Autodesk Inventor part; units mm, degrees
ref_plane "YZ Plane" through (0, 0, 0) normal (1, 0, 0) x (0, 1, 0)
ref_plane "XZ Plane" through (0, 0, 0) normal (0, 1, 0) x (-1, 0, 0)
ref_plane "XY Plane" through (0, 0, 0) normal (0, 0, 1) x (1, 0, 0)
sketch "Skizze1" plane through (0, 0, 0) normal (0, 0, 1) x (1, 0, 0)
  circle A0 centre (0.0001, -0.0022) radius 3.9802
  circle A1 centre (-8.37, 7.9978) radius 1.4
  circle A2 centre (8.3745, -8.0022) radius 1.4
  line L0 (-9.5383, 7.2264) -> (-3.2198, -2.3418)
  line L1 (-7.6522, 9.1998) -> (1.8915, 3.4999)
  line L2 (9.5428, -7.2307) -> (3.3215, 2.191)
  line L3 (-1.8517, -3.5253) -> (7.6567, -9.2041)
  point P0 (0, 0)
extrude "Extrusion1" add sketch "Skizze1" along normal blind 2
sketch "Skizze2" plane through (0, 0, 2) normal (0, 0, 1) x (1, 0, 0)
  arc A0 (-7.6522, 9.1998) -> (-9.5383, 7.2264) centre (-8.37, 7.9978) ccw
  line L0 (-9.5383, 7.2264) -> (-3.2198, -2.3418)
  arc A1 (-3.2198, -2.3418) -> (-1.8517, -3.5253) centre (0.0001, -0.0022) ccw
  line L1 (-1.8517, -3.5253) -> (7.6567, -9.2041)
  arc A2 (7.6567, -9.2041) -> (9.5428, -7.2307) centre (8.3745, -8.0022) ccw
  line L2 (9.5428, -7.2307) -> (3.3215, 2.191)
  arc A3 (3.3215, 2.191) -> (1.8915, 3.4999) centre (0.0001, -0.0022) ccw
  line L3 (1.8915, 3.4999) -> (-7.6522, 9.1998)
  arc A4 (-6.6267, 10.9169) -> (-11.2072, 6.1243) centre (-8.37, 7.9978) ccw
  line L4 (-11.2072, 6.1243) -> (-4.8666, -3.4774)
  arc A5 (-4.8666, -3.4774) -> (-2.8352, -5.2674) centre (0.0001, -0.0022) ccw
  line L5 (-2.8352, -5.2674) -> (6.6312, -10.9212)
  arc A6 (6.6312, -10.9212) -> (11.2118, -6.1287) centre (8.3745, -8.0022) ccw
  line L6 (11.2118, -6.1287) -> (4.9905, 3.2931)
  arc A7 (4.9905, 3.2931) -> (2.8837, 5.2369) centre (0.0001, -0.0022) ccw
  line L7 (2.8837, 5.2369) -> (-6.6267, 10.9169)
  point P0 (0, 0)
  dimension "d2" = 2
extrude "Extrusion2" add sketch "Skizze2" against normal up to surface (2 mm away)
sketch "Skizze3" plane through (0, 0, 2) normal (0, 0, 1) x (1, 0, 0)
  circle A0 centre (0.0001, -0.0022) radius 3.9802
  circle A1 centre (-8.37, 7.9978) radius 1.4
  circle A2 centre (8.3745, -8.0022) radius 1.4
  circle A3 centre (0.0001, -0.0022) radius 3.35
  point P0 (0, 0)
  dimension "d5" = 6.7
extrude "Extrusion3" cut sketch "Skizze3" against normal through all contours A1 | A2 | A3
sketch "Skizze4" plane through (0, 0, 2) normal (0, 0, 1) x (1, 0, 0)
  circle A0 centre (-8.37, 7.9978) radius 1.4
  circle A1 centre (8.3745, -8.0022) radius 1.4
  point P0 (0, 0)
hole "Bohrung1" at (-8.37, 7.9978, 2) at (8.3745, -8.0022, 2) direction (0, 0, -1) diameter 2.8 end through all
chamfer "Fase1" distance 1 angle 45 1 edges at (-3.3499, -0.0022, 2)
properties part number "IM_Lensholder_macroscope"
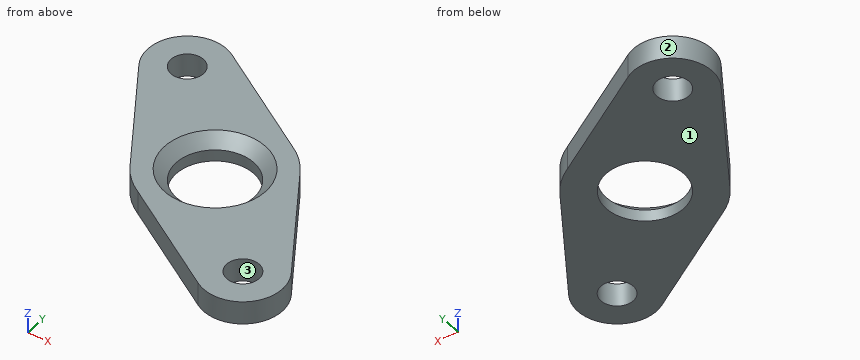
Could you check a few things on this model? Use its own coordinates, in mm. Face numbers are marked on the shaded views. Give positions to 0.01 mm unless a question says otherwise; leave off trailing zeros. Order: outer loops, then holes, each group sorted by start corner. A loop starts at its lowest first (then second) coordinate and runs counter-clockwise, first axis right, second up. Notation, with made-up numbers: (-29.75, 80.5) - (22.25, 80.5) arc R28 cw to (22.25, 119.5) - close; hole circle Ø6 at (31.25, 65). An arc over 180 degrees is marked (long way). Return JSON: item names as keys, results as strings. Group by question number.
Q1. Thinking about a two-plate mould opening in X: for the marked faces 1, 2 and 3, which applies, pulls with the +X half, pulls with the -X half, needs draft (parallel to the pull), parting line crosses it, or undercut?
Q2. Suppose I cut it at C-C, the plane x = -6. Please give me the cut outline in (y, z), and give its area (3 significant figures).
Q3. Suppose I cut it at D-D, the plane y = 5.5. Please give me the cut outline in (x, z).
Q4. Please list where these lines run through material, in increasing order: line 1 along Y through (x, z) = (2.5, 1.45); line 2 along X through (y, z) = (8.5, 0.85); line 3 along X through (y, z) = (3, 1.1). Write a range as [from, to].
Q5. Will these pins go through, and if not, where does the flat tip stop? pin 1 Ø3.5 at (x, y) = (8.37, -8) entering from -Z; pin 2 Ø1 at (y, z) = (7.5, 1.5) entering from +X.
Q6. Suppose I cut it at A-A, the plane z = 1.35. Please give me the cut outline in (x, y), and give its area (3 significant figures).
Q7. Suppose I cut it at B-B, the plane x = -8.37. Please give me the cut outline in (y, z).
Resolved:
{
 "1": {"face 1": "needs draft", "face 2": "parting line crosses it", "face 3": "undercut"},
 "2": {"outline": "(-1.76, 0) - (10.54, 0) - (10.54, 2) - (-1.76, 2) - close", "area": "24.6 mm2"},
 "3": {"outline": "(-10.79, 0) - (2.44, 0) - (2.44, 2) - (-10.79, 2) - close"},
 "4": {"line 1": "y = [-8.45, -2.86], [2.86, 5.47]", "line 2": "x = [-11.73, -9.68], [-7.06, -2.58]", "line 3": "x = [-9.14, -1.7], [1.7, 5.18]"},
 "5": {"pin 1": "stops at z = 0", "pin 2": "stops at x = -0.07"},
 "6": {"outline": "(-11.21, 6.12) - (-4.87, -3.48) arc R5.98 ccw to (-2.84, -5.27) - (6.63, -10.92) arc R3.4 ccw to (11.21, -6.13) - (4.99, 3.29) arc R5.98 ccw to (2.88, 5.24) - (-6.63, 10.92) arc R3.4 ccw to start; hole circle Ø2.8 at (-8.37, 8); hole circle Ø7.4 at (0, 0); hole circle Ø2.8 at (8.37, -8)", "area": "204 mm2"},
 "7": {"outline": "(1.83, 0) - (6.6, 0) - (6.6, 2) - (1.83, 2) - close; (9.4, 0) - (11.4, 0) - (11.4, 2) - (9.4, 2) - close"}
}
